Autodesk Inventor part; units mm, degrees
ref_plane "Work Plane1" through (2.75, 0, 0) normal (0, -1, 0) x (1, 0, 0)
ref_plane "YZ Plane" through (0, 0, 0) normal (1, 0, 0) x (0, 1, 0)
ref_plane "XZ Plane" through (0, 0, 0) normal (0, 1, 0) x (-1, 0, 0)
sketch "Skizze1" plane through (0, 0, 0) normal (0, 0, 1) x (1, 0, 0)
  line L0 (30, 4) -> (30, 0)
  line L1 (-12, 0) -> (30, 0)
  line L2 (-20.4, 0) -> (38.4, 0)
  line L3 (0, 4.8) -> (0, -0.8)
  line L4 (-12, 4) -> (-12, 0)
  line L5 (8, 4) -> (8, 0) construction
  line L6 (-20.4, 0) -> (38.4, 0)
  line L7 (-12, 4) -> (30, 4)
  dimension "d4" = 12
  dimension "d5" = 30
  dimension "d6" = 22
  dimension "d13" = 8
revolve "Körper" add sketch "Skizze1" angle 360 about axis through (-12, 0, 0) along (1, 0, 0)
thread "Gewinde1"
thread "Gewinde2"
chamfer "Fase1" distance 0.6145 distance2 0.6134 1 edges at (30, -4, 0) measured on face at (30, -0.0467, 2.2623)
chamfer "Fase2" distance 0.5423 distance2 0.6134 1 edges at (-12, -4, 0) measured on face at (15.591, 3.9482, -0.6416)
ref_plane "Work Plane1" through (2.75, 0, 0) normal (0, -1, 0) x (1, 0, 0)
equation "\"d4\" = KOH"
equation "\"d5\" = NLG"
equation "\"d6\" = GEL"
equation "\"d13\" = GD"
equation "\"d1\" = KOH"
equation "\"d7\" = GEL + GAL"
equation "\"d10\" = -0.5 * SPD + 0.5 * GD"
equation "\"d12\" = -0.5 * SPD + 0.5 * GD"
equation "\"NLG\" = 30"
equation "\"GEL\" = 22"
equation "\"GAL\" = 0.61345 * PTC"
equation "\"SPD\" = NND - 1.2269 * PTC"
equation "\"d0\" = GD"
equation "\"GUL\" = 0.61345 * PTC"
equation "\"KOH\" = 12"
equation "\"GD\" = NND"
equation "\"BDM\" = NND"
equation "\"GUL1\" = 0.54127"
equation "\"GAL1\" = GAL"
equation "\"d80\" = -GUL - GEL"
equation "\"d86\" = -KOH + GUL1"
equation "\"PTC\" = 1"
equation "\"THREADDIA\" = 8"
equation "\"TOA\" = 30deg"
equation "\"NND\" = 8"
equation "\"GD1\" = THREADDIA - 1.2269 * PTC"
properties part number "UNI 5910 - M8 x 1 x 30" material "Stahl, weich"
Model file for the job. Use its own axes, mm. Coordinates: 2 decimals unless noted, no trailing zeros. Loops run counter-clockwise (first coordinate to the right, second up) from the corner with the lowest first, then second, coordinate; pieces in that order, holes last. Notation, with made-up numbers: (72, -38) - (81, -38) arc R14 cw to (81, -18) - close; hole circle Ø8 at (18.25, 70). An arc over 180 degrees is marked (long way). Write item = value, one per line. Start each with the question number.
Item 1: Saw through at A-A, the plane x = 19. List the corners of the cut face in (y, z), then the cut area to 3 significant figures.
Item 2: Drop flat-ended pins along their axis: pin 1 Ø1 at (x, z) = (4.5, 1.5) entering from -Y; pin 2 Ø1 at (x, z) = (-4, -3) entering from -Y; pin 3 Ø3 at (x, y) = (13, 2) entering from +Z. Give the stop position or say it passes through.
Item 3: Wall check: probe 1 along Z at (x, y) = (10.5, -0.25); probe 2 along Z at (x, y) = (-7.5, 0.75). Give the ranges that are in metal, low to high. Write a range as [from, to].
Answers:
q1.outline = circle Ø8 at (0, 0)
q1.area = 50.3 mm2
q2.pin_1 = -3.87
q2.pin_2 = -3.12
q2.pin_3 = 3.97
q3.probe_1 = [-3.99, 3.99]
q3.probe_2 = [-3.93, 3.93]
